Read the model definition and answer for the solid it produces. Units are mm, in the model's axes. A direction names the side the tool comes from. Give positions to 0.01 mm unless a question says otherwise; leave off trailing zeros. Order: outer loops, then holes, each group sorted by start corner. A loop starts at its lowest first (then second) coordinate and runs counter-clockwise, first axis right, second up. Notation, with made-up numbers: (8, 5.5) -> (46, 5.5) arc R25 cw to (46, 41.5) -> close; hole circle Ø1 at (22.5, 34.25). An arc over 180 degrees is marked (long way). Answer as CSV lines item,"result". Start each with the question number.
1) Flat-ended cylindrical pins translate along their axes: pin 1 Ø1.8 at (x, y) = (0, 0) entering from -Z; pin 2 Ø0.9 at (x, z) = (-25.5, 1) entering from -Y; pin 3 Ø1.5 at (y, z) = (15, 1) entering from -X; pin 4 Ø2 at (x, y) = (0, 7.5) entering from -Z. Find the tip coordinate at first contact, or state that the pin passes through.
2) For faces 1 (the face through (-23.6, 15, 1)), 2 (the face through (2, 17.5, 1)), 3 (the face through (-25, -7.5, 1)), 4 (the face through (-25, -12.5, 1)), 5 (the face through (23.6, 10, 1)), determine the directions among +Z, -Z, +X, -X, +Y, -Y from which every point of the face is accessible in a straight line to the end or side of a thin tool.
3) Find section A-A (x = 0). Determine the outline of the cut face in (y, z).
4) Straight lines are drawn through the part: L1, parallel to Y at x = 0, z = 0.95; L2, parallel to X at y = 4, z = 1.55; L3, parallel to X at y = -5, z = 0.8. For each, find the intervals that lie inside material, in ascending order. Write a range as from..to.
5) The mould has two halves that part along X. Classify faces 6 (the face through (-26.6, 0, 1)), 7 (the face through (-25, 12.5, 1)), 8 (the face through (-0.163, -8.232, 1.521)): +X half, -X half, draft (parallel to the pull), parting line (faces both ways), or undercut.
6) Find section C-C (y = 3.75). Determine the outline of the cut face in (x, z), and give its area (3 significant figures).
7) Find section D-D (z = 2.5). State how many separate pieces and enclosed holes the cut face has, and give its area (3 significant figures).
8) Find section B-B (y = 0). Determine the outline of the cut face in (x, z).
```python
from build123d import *

# Parameters (mm, degrees)
SALIENTE_EXTRUIR1_DEPTH = 3
CORTAR_EXTRUIR1_REACH   = 33.981
CROQUIS2_R              = 0.75
CROQUIS2_R_2            = 1.5


with BuildPart() as part:
    # Croquis1 → Saliente-Extruir1 (new body)
    with BuildSketch(Plane.XY):
        Polygon((26.6, 2.5), (26.6, 7.5), (23.6, 7.5), (23.6, 12.5), (26.6, 12.5), (26.6, 17.5), (26.581338058, 17.5), (-23.6, 17.5), (-23.6, 12.5), (-26.6, 12.5), (-26.6, 7.5), (-23.6, 7.5), (-23.6, 2.5), (-26.6, 2.5), (-26.6, -2.5), (-23.6, -2.5), (-23.6, -7.5), (-26.6, -7.5), (-26.6, -12.5), (-23.6, -12.5), (-23.6, -17.5), (26.6, -17.5), (26.6, -12.5), (23.6, -12.5), (23.6, -7.5), (26.6, -7.5), (26.6, -2.5), (23.6, -2.5), (23.6, 2.5), align=None)
    extrude(amount=SALIENTE_EXTRUIR1_DEPTH)

    # Croquis2 → Cortar-Extruir1 (cut, up to next)
    with BuildSketch(Plane.XY.offset(3), mode=Mode.PRIVATE) as cortar_extruir1_sk1:
        with Locations((0, 7.5)):
            Circle(CROQUIS2_R)
    cortar_extruir1_tool1 = extrude(cortar_extruir1_sk1.sketch, amount=-CORTAR_EXTRUIR1_REACH, mode=Mode.PRIVATE) & part.part
    # Croquis2 → Cortar-Extruir1 (cut, up to next)
    with BuildSketch(Plane.XY.offset(3), mode=Mode.PRIVATE) as cortar_extruir1_sk2:
        with Locations((6.495190528, 3.75)):
            Circle(CROQUIS2_R)
    cortar_extruir1_tool2 = extrude(cortar_extruir1_sk2.sketch, amount=-CORTAR_EXTRUIR1_REACH, mode=Mode.PRIVATE) & part.part
    # Croquis2 → Cortar-Extruir1 (cut, up to next)
    with BuildSketch(Plane.XY.offset(3), mode=Mode.PRIVATE) as cortar_extruir1_sk3:
        with Locations((6.495190528, -3.75)):
            Circle(CROQUIS2_R)
    cortar_extruir1_tool3 = extrude(cortar_extruir1_sk3.sketch, amount=-CORTAR_EXTRUIR1_REACH, mode=Mode.PRIVATE) & part.part
    # Croquis2 → Cortar-Extruir1 (cut, up to next)
    with BuildSketch(Plane.XY.offset(3), mode=Mode.PRIVATE) as cortar_extruir1_sk4:
        with Locations((0, -7.5)):
            Circle(CROQUIS2_R)
    cortar_extruir1_tool4 = extrude(cortar_extruir1_sk4.sketch, amount=-CORTAR_EXTRUIR1_REACH, mode=Mode.PRIVATE) & part.part
    # Croquis2 → Cortar-Extruir1 (cut, up to next)
    with BuildSketch(Plane.XY.offset(3), mode=Mode.PRIVATE) as cortar_extruir1_sk5:
        with Locations((-6.495190528, -3.75)):
            Circle(CROQUIS2_R)
    cortar_extruir1_tool5 = extrude(cortar_extruir1_sk5.sketch, amount=-CORTAR_EXTRUIR1_REACH, mode=Mode.PRIVATE) & part.part
    # Croquis2 → Cortar-Extruir1 (cut, up to next)
    with BuildSketch(Plane.XY.offset(3), mode=Mode.PRIVATE) as cortar_extruir1_sk6:
        with Locations((-6.495190528, 3.75)):
            Circle(CROQUIS2_R)
    cortar_extruir1_tool6 = extrude(cortar_extruir1_sk6.sketch, amount=-CORTAR_EXTRUIR1_REACH, mode=Mode.PRIVATE) & part.part
    # Croquis2 → Cortar-Extruir1 (cut, up to next)
    with BuildSketch(Plane.XY.offset(3), mode=Mode.PRIVATE) as cortar_extruir1_sk7:
        Circle(CROQUIS2_R_2)
    cortar_extruir1_tool7 = extrude(cortar_extruir1_sk7.sketch, amount=-CORTAR_EXTRUIR1_REACH, mode=Mode.PRIVATE) & part.part
    add(cortar_extruir1_tool1.solids().sort_by_distance((0, 7.5, 3))[0], mode=Mode.SUBTRACT)
    add(cortar_extruir1_tool2.solids().sort_by_distance((6.495191, 3.75, 3))[0], mode=Mode.SUBTRACT)
    add(cortar_extruir1_tool3.solids().sort_by_distance((6.495191, -3.75, 3))[0], mode=Mode.SUBTRACT)
    add(cortar_extruir1_tool4.solids().sort_by_distance((0, -7.5, 3))[0], mode=Mode.SUBTRACT)
    add(cortar_extruir1_tool5.solids().sort_by_distance((-6.495191, -3.75, 3))[0], mode=Mode.SUBTRACT)
    add(cortar_extruir1_tool6.solids().sort_by_distance((-6.495191, 3.75, 3))[0], mode=Mode.SUBTRACT)
    add(cortar_extruir1_tool7.solids().sort_by_distance((0, 0, 3))[0], mode=Mode.SUBTRACT)


solid = part.part
```
Findings below:
1,pin 1,"through"
1,pin 2,"y = -12.5"
1,pin 3,"x = -23.6"
1,pin 4,"z = 0"
2,face 1,"+Z, -Z, -X, +Y"
2,face 2,"+Z, -Z, +X, -X, +Y"
2,face 3,"+Z, -Z, -X"
2,face 4,"+Z, -Z, -X, -Y"
2,face 5,"+Z, -Z, +X"
3,outline,"(-17.5, 0) -> (-8.25, 0) -> (-8.25, 3) -> (-17.5, 3) -> close; (-6.75, 0) -> (-1.5, 0) -> (-1.5, 3) -> (-6.75, 3) -> close; (1.5, 0) -> (6.75, 0) -> (6.75, 3) -> (1.5, 3) -> close; (8.25, 0) -> (17.5, 0) -> (17.5, 3) -> (8.25, 3) -> close"
4,L1,"-17.5..-8.25, -6.75..-1.5, 1.5..6.75, 8.25..17.5"
4,L2,"-23.6..-7.2, -5.79..5.79, 7.2..26.6"
4,L3,"-23.6..26.6"
5,face 6,"-X half"
5,face 7,"draft"
5,face 8,"undercut"
6,outline,"(-23.6, 0) -> (-7.25, 0) -> (-7.25, 3) -> (-23.6, 3) -> close; (-5.75, 0) -> (5.75, 0) -> (5.75, 3) -> (-5.75, 3) -> close; (7.25, 0) -> (26.6, 0) -> (26.6, 3) -> (7.25, 3) -> close"
6,area,"142 mm²"
7,separate pieces,"1"
7,enclosed holes,"7"
7,area,"1,740 mm²"
8,outline,"(-26.6, 0) -> (-1.5, 0) -> (-1.5, 3) -> (-26.6, 3) -> close; (1.5, 0) -> (23.6, 0) -> (23.6, 3) -> (1.5, 3) -> close"
